```python
from build123d import *

# Parameters (mm, degrees)
SKETCH2_OUTSIDE_W       = 164.146
SKETCH2_OUTSIDE_H       = 164.146
SKETCH2_OUTSIDE_W_2     = 105
SKETCH2_OUTSIDE_H_2     = 145.767420334
CUT_EXTRUDE2_DEPTH      = 116.381974501
BOSS_EXTRUDE2_REACH     = 112.568
SKETCH3_W               = 3.579145551
SKETCH3_H               = 65.962110336
BOSS_EXTRUDE4_DEPTH     = 150
CUT_EXTRUDE3_DEPTH      = 171.58815789
CUT_EXTRUDE3_DEPTH_BACK = 171.58815789
SKETCH5_W               = 112.520122243
SKETCH5_H               = 235.639617785
CUT_EXTRUDE4_DEPTH      = 171.587954009
CUT_EXTRUDE4_DEPTH_BACK = 171.587954009
SKETCH6_R               = 1.8


with BuildPart() as part:
    # Sketch1 → Revolve1 (revolve)
    with BuildSketch(Plane.XY):
        with BuildLine():
            Line((62, 0), (59, 0))
            ThreePointArc((59, 0), (42.363721251, 46.52102369), (0, 71.943189953))
            Line((0, 71.943189953), (0, 75))
            ThreePointArc((0, 75), (44.493217858, 48.65439343), (62, 0))
        make_face()
    revolve(axis=Axis((0, 75, 0), (0, -1, 0)))

    # Sketch2 outside → Cut-Extrude2 (cut, through all)
    with BuildSketch(Plane(origin=(0, 0, 0), x_dir=(-1, 0, 0), z_dir=(0, -1, 0))):
        Rectangle(SKETCH2_OUTSIDE_W, SKETCH2_OUTSIDE_H)
        Rectangle(SKETCH2_OUTSIDE_W_2, SKETCH2_OUTSIDE_H_2, mode=Mode.SUBTRACT)
    extrude(amount=-CUT_EXTRUDE2_DEPTH, mode=Mode.SUBTRACT)

    # Sketch3 → Boss-Extrude2 (add, up to next)
    with BuildSketch(Plane.XZ, mode=Mode.PRIVATE) as boss_extrude2_sk1:
        with Locations((-50.710427225, 0)):
            Rectangle(SKETCH3_W, SKETCH3_H)
    boss_extrude2_tool1 = extrude(boss_extrude2_sk1.sketch, amount=-BOSS_EXTRUDE2_REACH, mode=Mode.PRIVATE) - part.part
    # Sketch3 → Boss-Extrude2 (add, up to next)
    with BuildSketch(Plane.XZ, mode=Mode.PRIVATE) as boss_extrude2_sk2:
        with Locations((50.710427225, 0)):
            Rectangle(SKETCH3_W, SKETCH3_H)
    boss_extrude2_tool2 = extrude(boss_extrude2_sk2.sketch, amount=-BOSS_EXTRUDE2_REACH, mode=Mode.PRIVATE) - part.part
    add(boss_extrude2_tool1.solids().sort_by_distance((-50.710427, 0, 0))[0])
    add(boss_extrude2_tool2.solids().sort_by_distance((50.710427, 0, 0))[0])

    # Sketch4 → Boss-Extrude4 (add)
    with BuildSketch(Plane(origin=(0, 0, 0), x_dir=(-1, 0, 0), z_dir=(0, -1, 0))):
        with BuildLine():
            Line((52.500662853, -32.98), (48.921565797, -32.98))
            ThreePointArc((48.921565797, -32.98), (0, -59), (-48.921565797, -32.98))
            Line((-48.921565797, -32.98), (-52.500662853, -32.98))
            ThreePointArc((-52.500662853, -32.98), (0, -62), (52.500662853, -32.98))
        make_face()
        with BuildLine():
            Line((-48.921565797, 32.98), (-52.500662853, 32.98))
            ThreePointArc((-52.500662853, 32.98), (0, 62), (52.500662853, 32.98))
            Line((52.500662853, 32.98), (48.921565797, 32.98))
            ThreePointArc((48.921565797, 32.98), (0, 59), (-48.921565797, 32.98))
        make_face()
    extrude(amount=BOSS_EXTRUDE4_DEPTH)

    # Sketch5 → Cut-Extrude3 (cut, two sides: drawn at the far end of the back side and taken through both)
    with BuildSketch(Plane.XY.offset(-CUT_EXTRUDE3_DEPTH_BACK)):
        with Locations((-56.260061122, -36.450714171)):
            Rectangle(SKETCH5_W, SKETCH5_H)
    extrude(amount=CUT_EXTRUDE3_DEPTH + CUT_EXTRUDE3_DEPTH_BACK, mode=Mode.SUBTRACT)

    # Sketch6 → Cut-Extrude4 (cut, two sides: drawn at the far end of the back side and taken through both)
    with BuildSketch(Plane(origin=(52.5, 0, 0), x_dir=(0, 0, -1), z_dir=(1, 0, 0)).offset(-CUT_EXTRUDE4_DEPTH_BACK)):
        with Locations((-5, 10)):
            Circle(SKETCH6_R)
        with Locations((5, 10)):
            Circle(SKETCH6_R)
    extrude(amount=CUT_EXTRUDE4_DEPTH + CUT_EXTRUDE4_DEPTH_BACK, mode=Mode.SUBTRACT)


solid = part.part
```
Geometry: final body of the model. Coordinates: model frame, mm. A direction names the side the tool comes from. Coordinates: 2 decimals unless noted, no trailing zeros. Order: outer loops, then holes, each group sorted by start corner. A loop starts at its lowest first (then second) coordinate and runs counter-clockwise, first axis right, second up. Notation, with made-up numbers: M 6.25,72 L 48.25,72 A14 cw 48.25,81 Z; hole C -12.5,5 d1. An arc over 180 degrees is marked long. Answer in a Markdown table with one row per item. Add a question column.
Q1. Reachability of faces 1 (the cylindrical face through (27.35, -73.95, 52.28)), 2 (the flat face through (28, -150, 53)) from +Z, -Z, +X, -X, +Y, -Y: full face, straight path, thin tool, end or side. Return the list, or none.
Q2. Section query A-A on y = -72. Return the cut outline in (x, z).
Q3. Line query: L1, parallel to Z at x = 50.4, y = 10; L2, parallel to Z at x = 10, y = 0.5; L3, parallel to Z at x = 9, y = -113. Output: solid intervals per line, ascending.
Q4. Contact query for flat-ended pins moving along their axis: P1, Ø10, axis at x = 11, y = -84, coming from the -Z side; P2, Ø2, axis at x = 8, y = -21, coming from the +Z side; P3, Ø3, axis at x = 29.5, y = 48, coming from the +Z side; P4, Ø3, axis at y = 10, z = 5, coming from the -X side. Output: stop coordinate, or through.
Q5. Mould query, pull axis Z, two halves, no side actions, for faces 3 (the flat face through (28, -150, -53)), 4 (the cylindrical face through (30.377, -73.95, -54.049)), 5 (the flat face through (48.921, 14, 0)). Classes: released by +Z, released by -Z, zero draft, split by the parting line, or undercut.
Completed:
| question | item | result |
|---|---|---|
| 1 | face 1 | -X, -Y |
| 1 | face 2 | +Z, -Z, +X, -X, -Y |
| 2 | outline | M 0,-62 A62 ccw 52.5,-32.98 L 48.92,-32.98 A59 cw 0,-59 Z; M 0,59 A59 cw 48.92,32.98 L 52.5,32.98 A62 ccw 0,62 Z |
| 3 | L1 | z = -34.97 to -6.8, -3.2 to 3.2, 6.8 to 34.97 |
| 3 | L2 | z = -61.19 to -58.14, 58.14 to 61.19 |
| 3 | L3 | z = -61.34 to -58.31, 58.31 to 61.34 |
| 4 | P1 | stops at z = -61.71 |
| 4 | P2 | stops at z = 61.6 |
| 4 | P3 | stops at z = 36 |
| 4 | P4 | passes through |
| 5 | face 3 | zero draft |
| 5 | face 4 | released by -Z |
| 5 | face 5 | undercut |
